Geometry: final body of the model. Coordinates: model frame, mm. Face numbers are marked on the shaded views. A direction names the side the tool comes from. Round coordinates to 2 decimals unless told otherwise and drop trailing zeros. Loops run counter-clockwise (first coordinate to the right, second up) from the corner with the lowest first, then second, coordinate; pieces in that order, holes last. Notation, with made-up numbers: M 50.25,-28 L 79.25,-28 A20 ccw 79.25,-18 Z; hole C 46.25,89 d3. An arc over 180 degrees is marked long. Write each question's results on one line, items separated by ' | '.
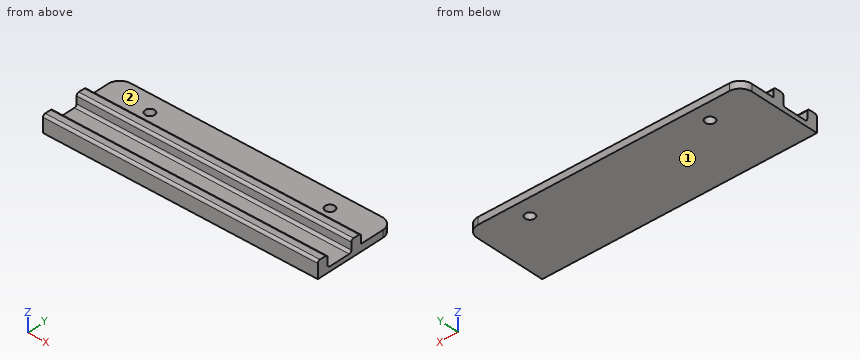
```python
from build123d import *

# Parameters (mm, degrees)
SKETCH1_W           = 116
SKETCH1_H           = 20
BOSS_EXTRUDE1_DEPTH = 2
SKETCH2_W           = 116
SKETCH2_H           = 4.5
BOSS_EXTRUDE2_DEPTH = 5
FILLET1_R           = 1
SKETCH3_W           = 116
SKETCH3_H           = 3
BOSS_EXTRUDE3_DEPTH = 15
FILLET2_R           = 5
SKETCH4_R           = 2
CUT_EXTRUDE1_DEPTH  = 15


with BuildPart() as part:
    # Sketch1 → Boss-Extrude1 (new body)
    with BuildSketch(Plane.XY):
        with Locations((58, 10)):
            Rectangle(SKETCH1_W, SKETCH1_H)
    extrude(amount=BOSS_EXTRUDE1_DEPTH)

    # Sketch2 → Boss-Extrude2 (add)
    with BuildSketch(Plane.XY.offset(2)):
        with Locations((58, 17.75)):
            Rectangle(SKETCH2_W, SKETCH2_H)
        with Locations((58, 2.25)):
            Rectangle(SKETCH2_W, SKETCH2_H)
    extrude(amount=BOSS_EXTRUDE2_DEPTH)

    # Fillet1
    fillet1_edges = [part.edges().sort_by_distance(p)[0] for p in [
        (58, 15.5, 2),
        (58, 15.5, 7),
        (58, 20, 7),
        (58, 4.5, 2),
        (58, 0, 7),
        (58, 4.5, 7),
    ]]
    fillet(fillet1_edges, radius=FILLET1_R)

    # Sketch3 → Boss-Extrude3 (add)
    with BuildSketch(Plane(origin=(0, 20, 0), x_dir=(1, 0, 0), z_dir=(0, 1, 0))):
        with Locations((58, -1.5)):
            Rectangle(SKETCH3_W, SKETCH3_H)
    extrude(amount=BOSS_EXTRUDE3_DEPTH)

    # Fillet2
    fillet2_edges = [part.edges().sort_by_distance(p)[0] for p in [
        (0, 35, 1.5),
        (116, 35, 1.5),
    ]]
    fillet(fillet2_edges, radius=FILLET2_R)

    # Sketch4 → Cut-Extrude1 (cut)
    with BuildSketch(Plane.XY.offset(3)):
        with Locations((96, 27.5)):
            Circle(SKETCH4_R)
        with Locations(Location((20, 27.5, 0), (0, 0, 180))):
            Circle(SKETCH4_R)
    extrude(amount=-CUT_EXTRUDE1_DEPTH, mode=Mode.SUBTRACT)


solid = part.part
```
1. Ray query, probe 1 along Y at (x, z) = (20, 1.2); probe 2 along Y at (x, z) = (96, 4); probe 3 along Y at (x, z) = (20, 2.3). Return the intervals inside material, ascending.
Answer key:
probe 1: y = 0 to 25.5, 29.5 to 35 | probe 2: y = 0 to 4.5, 15.5 to 20 | probe 3: y = 0 to 4.79, 15.21 to 25.5, 29.5 to 35
2. Section B-B (x = 20). Output: boundary loops of the cut face in (y, z), then the cut area to 3 significant figures.
Answer key:
outline: M 0,0 L 25.5,0 L 25.5,3 L 20,3 L 20,6 A1 ccw 19,7 L 16.5,7 A1 ccw 15.5,6 L 15.5,3 A1 cw 14.5,2 L 5.5,2 A1 cw 4.5,3 L 4.5,6 A1 ccw 3.5,7 L 1,7 A1 ccw 0,6 Z; M 29.5,0 L 35,0 L 35,3 L 29.5,3 Z | area: 118 mm²
3. Section A-A (z = 4.75). Output: boundary loops of the cut face in (x, y), then the cut area to 3 significant figures.
Answer key:
outline: M 0,0 L 116,0 L 116,4.5 L 0,4.5 Z; M 0,15.5 L 116,15.5 L 116,20 L 0,20 Z | area: 1,040 mm²
4. Section C-C (y = 27.5). Output: boundary loops of the cut face in (x, z).
Answer key:
outline: M 0,0 L 18,0 L 18,3 L 0,3 Z; M 22,0 L 94,0 L 94,3 L 22,3 Z; M 98,0 L 116,0 L 116,3 L 98,3 Z
5. Pin query (flat end, axial travel): P1, Ø1, axis at x = 42, y = 16.5, coming from the -Z side; P2, Ø4.5, axis at x = 74.5, y = 28, coming from the +Z side; P3, Ø1, axis at x = 45, z = 6, coming from the +Y side; P4, Ø7, axis at x = 79.5, y = 9, coming from the +Z side. Return the tip coordinate at first contact, or that it passes through.
Answer key:
P1: stops at z = 0 | P2: stops at z = 3 | P3: stops at y = 20 | P4: stops at z = 2
6. Section D-D (x = 35.5). Output: boundary loops of the cut face in (y, z), then the cut area to 3 significant figures.
Answer key:
outline: M 0,0 L 35,0 L 35,3 L 20,3 L 20,6 A1 ccw 19,7 L 16.5,7 A1 ccw 15.5,6 L 15.5,3 A1 cw 14.5,2 L 5.5,2 A1 cw 4.5,3 L 4.5,6 A1 ccw 3.5,7 L 1,7 A1 ccw 0,6 Z | area: 130 mm²
7. Access query for the marked faces 1 and 2. Directions: +Z, -Z, +X, -X, +Y, -Y. A direction counts if a zero-diameter tool reaches every point of the face in a straight line with its end or side. Return the directions, or none.
Answer key:
face 1: -Z, +X, -X, +Y, -Y | face 2: +Z, +X, -X, +Y
